from build123d import *
from build123d import SkipClean  # not in build123d's __all__

# Parameters (mm, degrees)
F0_W      = 70
F0_H      = 20
F1_DEPTH  = 1
F3_D      = 3
F4_R      = 5
F7_DEPTH  = 0.5
F9_DEPTH  = 69.001
F10_W     = 16
F10_H     = 9.25
F10_H_2   = 1.5
F11_DEPTH = 6.9
F12_R     = 1.9
F13_DEPTH = 4.5
F14_R     = 2
F15_DEPTH = 4
F16_R     = 1.5
F17_DEPTH = 1
F18_R     = 1.4
F19_DEPTH = 14.8


with BuildPart() as f1:
    # F0 (on Top) → F1 (new body)
    with BuildSketch(Plane.XY):
        Rectangle(F0_W, F0_H)
    extrude(amount=F1_DEPTH)

    # F3 (through all)
    with Locations(Plane.XY.offset(1)):
        with Locations((-28, 0), (28, 0)):
            Hole(F3_D / 2)

    # F4
    f4_edges = [f1.edges().sort_by_distance(p)[0] for p in [
        (-35, 10, 0.5),
        (-35, -10, 0.5),
        (35, 10, 0.5),
        (35, -10, 0.5),
    ]]
    fillet(f4_edges, radius=F4_R)

    # F5 (on face) + F6 (on face) → F7 (join)
    with BuildSketch(Plane.XY.offset(1)):
        with BuildLine():
            Line((-29.2990381057, 0.75), (-34, 0.75))
            Line((-34, 0.75), (-34, -0.75))
            Line((-34, -0.75), (-29.2990381057, -0.75))
            ThreePointArc((-29.2990381057, -0.75), (-29.5, 0), (-29.2990381057, 0.75))
        make_face()
        with BuildLine():
            Line((-22, 0.75), (-26.7009618943, 0.75))
            ThreePointArc((-26.7009618943, 0.75), (-26.5511112606, 0.3882285677), (-26.5, 0))
            ThreePointArc((-26.5, 0), (-26.5511112606, -0.3882285677), (-26.7009618943, -0.75))
            Line((-26.7009618943, -0.75), (-22, -0.75))
            Line((-22, -0.75), (-22, 0.75))
        make_face()
    with BuildSketch(Plane.XY.offset(1)):
        with BuildLine():
            Line((26.7009618943, 0.75), (22, 0.75))
            Line((22, 0.75), (22, -0.75))
            Line((22, -0.75), (26.7009618943, -0.75))
            ThreePointArc((26.7009618943, -0.75), (26.5, 0), (26.7009618943, 0.75))
        make_face()
        with BuildLine():
            Line((34, 0.75), (29.2990381057, 0.75))
            ThreePointArc((29.2990381057, 0.75), (29.4488887394, 0.3882285677), (29.5, 0))
            ThreePointArc((29.5, 0), (29.4488887394, -0.3882285677), (29.2990381057, -0.75))
            Line((29.2990381057, -0.75), (34, -0.75))
            Line((34, -0.75), (34, 0.75))
        make_face()
    with SkipClean():  # cleaning this boolean's faces spoils the solid; the shape is the same uncleaned
        extrude(amount=F7_DEPTH)

    # F8 (on face) → F9 (cut, through all)
    with BuildSketch(Plane(origin=(-34, 0, 0), x_dir=(0, -1, 0), z_dir=(-1, 0, 0))):
        Polygon((-0.75, 1.5), (-0.75, 1), (0, 1.5), align=None)
        Polygon((0.75, 1.5), (0, 1.5), (0.75, 1), align=None)
    with SkipClean():  # cleaning this boolean's faces spoils the solid; the shape is the same uncleaned
        extrude(amount=-F9_DEPTH, mode=Mode.SUBTRACT)

    # F10 (on face) → F11 (join)
    with BuildSketch(Plane.XY.offset(1)):
        with Locations((0, -5.375)):
            Rectangle(F10_W, F10_H)
        Rectangle(F10_W, F10_H_2)
        with Locations((0, 5.375)):
            Rectangle(F10_W, F10_H)
    with SkipClean():  # cleaning this boolean's faces spoils the solid; the shape is the same uncleaned
        extrude(amount=F11_DEPTH)

    # F12 (on face) → F13 (cut)
    with BuildSketch(Plane.XY.offset(7.9)):
        with Locations((-3.5, 5)):
            Circle(F12_R)
        with Locations((3.5, 5)):
            Circle(F12_R)
    with SkipClean():  # cleaning this boolean's faces spoils the solid; the shape is the same uncleaned
        extrude(amount=-F13_DEPTH, mode=Mode.SUBTRACT)

    # F14 (on face) → F15 (join)
    with BuildSketch(Plane.XY.offset(7.9)):
        with Locations((-3.5, -5)):
            Circle(F14_R)
        with Locations((3.5, -5)):
            Circle(F14_R)
    with SkipClean():  # cleaning this boolean's faces spoils the solid; the shape is the same uncleaned
        extrude(amount=F15_DEPTH)

    # F16 (on face) → F17 (join)
    with BuildSketch(Plane.XY.offset(1)):
        with Locations((-28, 0)):
            Circle(F16_R)
    with SkipClean():  # cleaning this boolean's faces spoils the solid; the shape is the same uncleaned
        extrude(amount=-F17_DEPTH)

    # F18 (on face) → F19 (join)
    with BuildSketch(Plane.XY.offset(1)):
        with Locations((-28, 0)):
            Circle(F18_R)
    with SkipClean():  # cleaning this boolean's faces spoils the solid; the shape is the same uncleaned
        extrude(amount=F19_DEPTH)


solid = f1.part
Here's how the part is built. I have some questions about the finished solid (model axes, mm). A direction names the side the tool comes from. Round coordinates to 2 decimals unless told otherwise and drop trailing zeros. Loops run counter-clockwise (first coordinate to the right, second up) from the corner with the lowest first, then second, coordinate; pieces in that order, holes last. Notation, with made-up numbers: (-29, 40) - (17, 40) arc R11 cw to (17, 49) - close; hole circle Ø1 at (3.5, 50.5). An arc over 180 degrees is marked (long way). One line per question, with ' | ' between items. Start each with the question number.
Q1. Please list where these lines run through material, in increasing order: line 1 (Y direction, x = 28, z = 0.5); line 2 (Y direction, x = -3.5, z = 4.35); line 3 (Z direction, x = 15, y = 0.25). Write a range as [from, to].
Q2. I want a section at A-A (z = 5.25). Write out the boundary of the cut face in (x, y), then the cut area to 3 significant figures.
Q3. Will these pins go through, and if not, where does the flat tip stop? pin 1 (3.5 mm diameter, centred on y = 2, z = 5, fed in from +X); pin 2 (5 mm diameter, centred on x = -0.5, y = -0.5, fed in from +Z); pin 3 (1 mm diameter, centred on x = -18.5, y = -3, fed in from +Z).
Q4. We'd pull the mould along Y, two halves only. Please class faces 3 (the flat face through (0, 0, 7.9)), 4 (the flat face through (3, 5, 3.4)), 5 (the flat face through (0, -10, 3)), 6 (the cylindrical face through (3.253, 6.884, 5.682)): +Y half, -Y half, draft (parallel to the pull), parting line (faces both ways), or undercut.
Q5. For faces 1 (the cylindrical face through (-5.1, -6.2, 9.9)), 2 (the flat face through (0, 10, 3)), which set-ups out of +Z, -Z, +X, -X, +Y, -Y let a thin tool reach every point of the face, with its end or its side?
Q6. I want a section at B-B (x = 28). Write out the boundary of the cut face in (y, z), then the cut area to 3 significant figures.
Q7. I want a section at D-D (z = 2.25). Write out the boundary of the cut face in (x, y).
Q8. I want a section at C-C (x = -23). Write out the boundary of the cut face in (y, z).
Response values:
1) line 1: y = [-10, -1.5], [1.5, 10] | line 2: y = [-10, 3.1], [6.9, 10] | line 3: z = [0, 1]
2) outline: circle Ø2.8 at (-28, 0); (-8, -10) - (8, -10) - (8, 10) - (-8, 10) - close; hole circle Ø3.8 at (-3.5, 5); hole circle Ø3.8 at (3.5, 5) | area: 303 mm²
3) pin 1: stops at x = 8 | pin 2: stops at z = 7.9 | pin 3: stops at z = 1
4) face 3: draft | face 4: undercut | face 5: -Y half | face 6: undercut
5) face 1: +Z | face 2: +Z, -Z, +X, -X, +Y
6) outline: (-10, 0) - (-1.5, 0) - (-1.5, 1) - (-10, 1) - close; (1.5, 0) - (10, 0) - (10, 1) - (1.5, 1) - close | area: 17.0 mm²
7) outline: circle Ø2.8 at (-28, 0); (-8, -10) - (8, -10) - (8, 10) - (-8, 10) - close
8) outline: (-10, 0) - (10, 0) - (10, 1) - (0.75, 1) - (0, 1.5) - (-0.75, 1) - (-10, 1) - close
